Check sheet for the modelled part. Datum: model origin and axes. Units: mm. A direction names the side the tool comes from. Give positions to 0.01 mm unless a question says otherwise; leave off trailing zeros. Write each loop counter-clockwise with the first axis right and the second up, starting at its lowest first coordinate (ties: lowest second). Pieces come first, ordered by that corner, then holes. Notation, with made-up numbers: (54, -21) -> (65, -21) arc R29 ccw to (65, 6) -> close; hole circle Ø6 at (-34, 82.5). An arc over 180 degrees is marked (long way). Use a Markdown table: item, result. Add a question column.
1. Scan lines: probe 1 along Z at (x, y) = (4.75, -4.4); probe 2 along X at (y, z) = (-2.75, 2.25); probe 3 along X at (y, z) = (-3.6, 1). Record each from-to range of solid material in increasing order. Write a range as [from, to].
2. Gauge pin test, flat ends, axial feed: P1, Ø2.5, axis at y = -3.5, z = 2, coming from the +X side; P2, Ø1.5, axis at x = 1.5, y = -3.5, coming from the -Z side. Record the tip position at first contact, or that the pin passes through.
3. Cross-section at D-D (z = 9). Enter the section's corners in (x, y).
4. Release check for a two-part mould opening along X. For faces 1 (the flat face through (2, 0, 6)), 2 (the flat face through (0, -2, 2)), 3 (the cylindrical face through (-3, -3, 9)) record: released by +X, released by -X, zero draft, split by the parting line, or undercut.
5. Set-up check for faces 4 (the cylindrical face through (9, -3, 8)), 5 (the flat face through (5, -2, 3)): record each of +Z, -Z, +X, -X, +Y, -Y from which the full face is reachable in a straight line by a thin tool's end or side.
6. Cross-section at A-A (z = 3.75). Enter the section's corners in (x, y).
7. Cross-section at C-C (x = 4.25). Enter the section's corners in (y, z).
from build123d import *

# Parameters (mm, degrees)
F1_DEPTH = 5
F2_R     = 4.99999


# Not quite as in the source:
# - a fillet or chamfer is up to 0.001 mm smaller than in the source, because OpenCascade refuses the exact size


with BuildPart() as f1:
    # F0 (on Front) → F1 (new body)
    with BuildSketch(Plane.XZ):
        Polygon((-5, 0), (0, 0), (0, 5), (5, 5), (5, 0), (10, 0), (10, 10), (-5, 10), align=None)
    extrude(amount=F1_DEPTH)

    # F2 (radius 5 in the source; OpenCascade refuses exactly that, so slightly less here)
    f2_edges = [f1.edges().sort_by_distance(p)[0] for p in [
        (10, -2.5, 10),
        (10, -2.5, 0),
        (-5, -2.5, 10),
        (-5, -2.5, 0),
    ]]
    fillet(f2_edges, radius=F2_R)


solid = f1.part
Worked answers:
| question | item | result |
|---|---|---|
| 1 | probe 1 | z = [5, 10] |
| 1 | probe 2 | x = [-4.18, 0], [5, 9.18] |
| 1 | probe 3 | x = [-3, 0], [5, 8] |
| 2 | P1 | stops at x = 9.68 |
| 2 | P2 | stops at z = 5 |
| 3 | outline | (-3, -5) -> (8, -5) -> (8, 0) -> (-3, 0) -> close |
| 4 | face 1 | zero draft |
| 4 | face 2 | undercut |
| 4 | face 3 | released by -X |
| 5 | face 4 | +Z, +X, +Y, -Y |
| 5 | face 5 | -Z, +Y, -Y |
| 6 | outline | (-4.84, -5) -> (0, -5) -> (0, 0) -> (-4.84, 0) -> close; (5, -5) -> (9.84, -5) -> (9.84, 0) -> (5, 0) -> close |
| 7 | outline | (-5, 5) -> (0, 5) -> (0, 10) -> (-5, 10) -> close |
